Read the model definition and answer for the solid it produces. Units are mm, in the model's axes. Face numbers are marked on the shaded views. A direction names the side the tool comes from. Give positions to 0.01 mm unless a question says otherwise; leave off trailing zeros. Loops run counter-clockwise (first coordinate to the right, second up) from the corner with the lowest first, then second, coordinate; pieces in that order, holes last. Notation, with made-up numbers: (38, 31.5) - (48, 31.5) arc R25 cw to (48, 61.5) - close; hole circle Ø11 at (82, -4). An arc over 180 degrees is marked (long way). Write item = value, one per line. Start each with the question number.
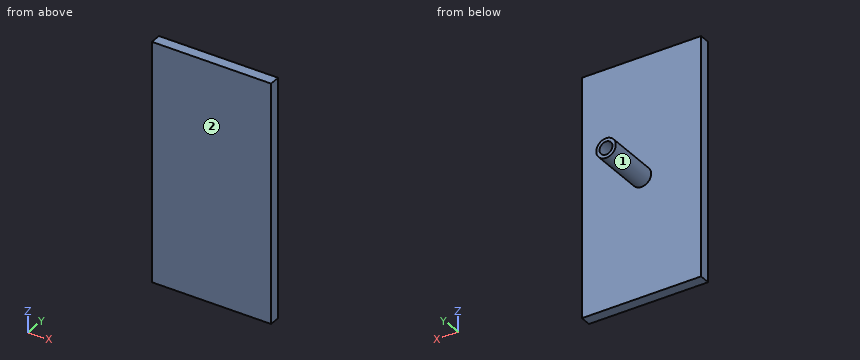
from build123d import *

# Parameters (mm, degrees)
SKETCH1_W           = 55
SKETCH1_H           = 110
BOSS_EXTRUDE3_DEPTH = 5
SKETCH3_R           = 4.5
BOSS_EXTRUDE4_DEPTH = 25
SKETCH4_R           = 3
CUT_EXTRUDE1_DEPTH  = 20


with BuildPart() as part:
    # Sketch1 → Boss-Extrude3 (new body)
    with BuildSketch(Plane(origin=(0, 0, 0), x_dir=(1, 0, 0), z_dir=(0, 1, 0))):
        with Locations((27.5, 55)):
            Rectangle(SKETCH1_W, SKETCH1_H)
    extrude(amount=BOSS_EXTRUDE3_DEPTH)

    # Sketch3 → Boss-Extrude4 (add)
    with BuildSketch(Plane(origin=(0, 5, 0), x_dir=(1, 0, 0), z_dir=(0, 1, 0))):
        with Locations((27.5, 55)):
            Circle(SKETCH3_R)
    extrude(amount=BOSS_EXTRUDE4_DEPTH)

    # Sketch4 → Cut-Extrude1 (cut)
    with BuildSketch(Plane(origin=(0, 30, 0), x_dir=(1, 0, 0), z_dir=(0, 1, 0))):
        with Locations((27.5, 55)):
            Circle(SKETCH4_R)
    extrude(amount=-CUT_EXTRUDE1_DEPTH, mode=Mode.SUBTRACT)


solid = part.part
1. A cutting plane is placed at C-C on y = 23.5. Give the vertices of the cut face in (x, z).
2. A cutting plane is placed at B-B on x = 27.5. Give the vertices of the cut face in (y, z), and give its area (3 significant figures).
3. A cutting plane is placed at D-D on y = 6.75. Give the vertices of the cut face in (x, z).
4. A cutting plane is placed at A-A on z = -55. Give the vertices of the cut face in (x, y).
5. A tool of negligible diameter and unlimited length cuts with its end or side. For the marked faces 1 and 2, from which of +Z, -Z, +X, -X, +Y, -Y can it reach the whole face along a straight path? Write none if from no direction.
6. Given P1, Ø1.5, axis at x = 41, z = -14.5, coming from the +Y side; P2, Ø3, axis at x = 26.5, z = -31.5, coming from the -Y side; P3, Ø5.5, axis at x = 27.5, z = -55, coming from the +Y side, each flat-ended and moving along its own axis, determine where each tip first touches the part or whether it passes through.
7. Consider line 1 along X through (y, z) = (17, -55); line 2 along Z through (x, y) = (27.5, 22); line 3 along Y through (x, z) = (13.5, -53.5). Determine where each line is inside the solid, lowest interval first. Write a range as [from, to].
Reply:
q1.outline = circle Ø9 at (27.5, -55); hole circle Ø6 at (27.5, -55)
q2.outline = (0, -110) - (5, -110) - (5, -59.5) - (30, -59.5) - (30, -58) - (10, -58) - (10, -52) - (30, -52) - (30, -50.5) - (5, -50.5) - (5, 0) - (0, 0) - close
q2.area = 655 mm^2
q3.outline = circle Ø9 at (27.5, -55)
q4.outline = (0, 0) - (55, 0) - (55, 5) - (32, 5) - (32, 30) - (30.5, 30) - (30.5, 10) - (24.5, 10) - (24.5, 30) - (23, 30) - (23, 5) - (0, 5) - close
q5.face_1 = +Y
q5.face_2 = +Z, -Z, +X, -X, -Y
q6.P1 = 5
q6.P2 = 0
q6.P3 = 10
q7.line_1 = [23, 24.5], [30.5, 32]
q7.line_2 = [-59.5, -58], [-52, -50.5]
q7.line_3 = [0, 5]
